```python
from build123d import *

# Parameters (mm, degrees)
F1_DEPTH = 8
F3_DEPTH = 25


with BuildPart() as f1:
    # F0 (on Top) → F1 (new body)
    with BuildSketch(Plane.XY):
        Polygon((20.7106781187, -50), (50, -20.7106781187), (50, 20.7106781187), (20.7106781187, 50), (-20.7106781187, 50), (-50, 20.7106781187), (-50, -20.7106781187), (-20.7106781187, -50), align=None)
    extrude(amount=F1_DEPTH)

    # F2 (on face) → F3 (cut)
    with BuildSketch(Plane.XY.offset(8)):
        with BuildLine():
            ThreePointArc((24.5349567524, 31.5917061451), (24.7489552671, 24.7485194141), (31.5921382283, 24.5344003832))
            ThreePointArc((31.5921382283, 24.5344003832), (28.2845203052, 28.2840221875), (24.5349567524, 31.5917061451))
        make_face()
        with BuildLine():
            ThreePointArc((24.5349567524, 31.5917061451), (28.2845203052, 28.2840221875), (31.5921382283, 24.5344003832))
            ThreePointArc((31.5921382283, 24.5344003832), (32.8418270546, 26.2270936053), (33.2845203052, 28.2840221875))
            ThreePointArc((33.2845203052, 28.2840221875), (30.052595846, 32.9609772741), (24.5349567524, 31.5917061451))
        make_face()
        with BuildLine():
            ThreePointArc((-4.9902248196, 39.6875), (0, 35), (4.9902248196, 39.6875))
            ThreePointArc((4.9902248196, 39.6875), (0, 40), (-4.9902248196, 39.6875))
        make_face()
        with BuildLine():
            ThreePointArc((-4.9902248196, 39.6875), (0, 40), (4.9902248196, 39.6875))
            ThreePointArc((4.9902248196, 39.6875), (4.9975556074, 39.8436735754), (5, 40))
            ThreePointArc((5, 40), (-0.1563264246, 44.9975556074), (-4.9902248196, 39.6875))
        make_face()
        with BuildLine():
            ThreePointArc((-31.5918062772, 24.5348278197), (-28.2841376224, 28.2844048719), (-24.5345293173, 31.5920380979))
            ThreePointArc((-24.5345293173, 31.5920380979), (-31.8196548252, 31.8199554809), (-31.5918062772, 24.5348278197))
        make_face()
        with BuildLine():
            ThreePointArc((-23.2841376224, 28.2844048719), (-23.607170575, 30.0524487732), (-24.5345293173, 31.5920380979))
            ThreePointArc((-24.5345293173, 31.5920380979), (-28.2841376224, 28.2844048719), (-31.5918062772, 24.5348278197))
            ThreePointArc((-31.5918062772, 24.5348278197), (-26.2272398702, 23.7270842076), (-23.2841376224, 28.2844048719))
        make_face()
        with BuildLine():
            ThreePointArc((-39.6875, -4.9902248196), (-40, 0), (-39.6875, 4.9902248196))
            ThreePointArc((-39.6875, 4.9902248196), (-45, 0), (-39.6875, -4.9902248196))
        make_face()
        with BuildLine():
            ThreePointArc((-35, 0), (-36.3556550657, 3.4232659844), (-39.6875, 4.9902248196))
            ThreePointArc((-39.6875, 4.9902248196), (-40, 0), (-39.6875, -4.9902248196))
            ThreePointArc((-39.6875, -4.9902248196), (-36.3556550657, -3.4232659844), (-35, 0))
        make_face()
        with BuildLine():
            ThreePointArc((-31.5921382283, -24.5344003832), (-31.8200853434, -31.8195249609), (-24.5349567524, -31.5917061451))
            ThreePointArc((-24.5349567524, -31.5917061451), (-28.2845203052, -28.2840221875), (-31.5921382283, -24.5344003832))
        make_face()
        with BuildLine():
            ThreePointArc((-31.5921382283, -24.5344003832), (-28.2845203052, -28.2840221875), (-24.5349567524, -31.5917061451))
            ThreePointArc((-24.5349567524, -31.5917061451), (-23.6075652186, -30.0520977283), (-23.2845203052, -28.2840221875))
            ThreePointArc((-23.2845203052, -28.2840221875), (-26.227591723, -23.7267154382), (-31.5921382283, -24.5344003832))
        make_face()
        with BuildLine():
            ThreePointArc((-4.9902248196, -39.6875), (0, -40), (4.9902248196, -39.6875))
            ThreePointArc((4.9902248196, -39.6875), (0, -35), (-4.9902248196, -39.6875))
        make_face()
        with BuildLine():
            ThreePointArc((5, -40), (4.9975556074, -39.8436735754), (4.9902248196, -39.6875))
            ThreePointArc((4.9902248196, -39.6875), (0, -40), (-4.9902248196, -39.6875))
            ThreePointArc((-4.9902248196, -39.6875), (-0.1563264246, -44.9975556074), (5, -40))
        make_face()
        with BuildLine():
            ThreePointArc((24.5344003832, -31.5921382283), (28.2840221875, -28.2845203052), (31.5917061451, -24.5349567524))
            ThreePointArc((31.5917061451, -24.5349567524), (24.7485194141, -24.7489552671), (24.5344003832, -31.5921382283))
        make_face()
        with BuildLine():
            ThreePointArc((33.2840221875, -28.2845203052), (32.8413470491, -26.2276318527), (31.5917061451, -24.5349567524))
            ThreePointArc((31.5917061451, -24.5349567524), (28.2840221875, -28.2845203052), (24.5344003832, -31.5921382283))
            ThreePointArc((24.5344003832, -31.5921382283), (30.052056545, -32.9614909605), (33.2840221875, -28.2845203052))
        make_face()
        with BuildLine():
            ThreePointArc((39.6875, -4.9902248196), (39.9217985567, -2.5), (40, 0))
            ThreePointArc((40, 0), (39.9217985567, 2.5), (39.6875, 4.9902248196))
            ThreePointArc((39.6875, 4.9902248196), (35, 0), (39.6875, -4.9902248196))
        make_face()
        with BuildLine():
            ThreePointArc((39.6875, 4.9902248196), (39.9217985567, 2.5), (40, 0))
            ThreePointArc((40, 0), (39.9217985567, -2.5), (39.6875, -4.9902248196))
            ThreePointArc((39.6875, -4.9902248196), (43.4232659844, -3.6443449343), (45, 0))
            ThreePointArc((45, 0), (43.4232659844, 3.6443449343), (39.6875, 4.9902248196))
        make_face()
    extrude(amount=-F3_DEPTH, mode=Mode.SUBTRACT)


solid = f1.part
```
Verification items for the finished model (mm, model axes). Round coordinates to 2 decimals unless told otherwise and drop trailing zeros. Loops run counter-clockwise (first coordinate to the right, second up) from the corner with the lowest first, then second, coordinate; pieces in that order, holes last. Notation, with made-up numbers: (25.5, 37) -> (68.5, 37) arc R5 cw to (68.5, 44) -> close; hole circle Ø6 at (89, 19.25). An arc over 180 degrees is marked (long way). Answer as a JSON object with one key per item and string values.
Q1. Go/stop test with a flat-tipped pin: P1, Ø2, axis at x = 19.5, y = 25, coming from the -Z side. Record where the tip stops, or that it passes through.
Data:
{"P1": "stops at z = 0"}
Q2. Section check C-C (z = 3). State how many separate pieces and enclosed holes the cut face has, then the cut area to 3 significant figures.
Data:
{"separate pieces": "1", "enclosed holes": "8", "area": "7,660 mm2"}
Q3. Draft check along X on faces 1 (the flat face through (-50, 0, 4)), 2 (the flat face through (0, -50, 4)), 3 (the flat face through (50, 0, 4)). Enter one of: pulls with the +X half, pulls with the -X half, needs draft (parallel to the pull), parting line crosses it, or undercut.
Data:
{"face 1": "pulls with the -X half", "face 2": "needs draft", "face 3": "pulls with the +X half"}
Q4. Section check A-A (x = 0). Record the boundary of the cut face in (y, z).
Data:
{"outline": "(-50, 0) -> (-45, 0) -> (-45, 8) -> (-50, 8) -> close; (-35, 0) -> (35, 0) -> (35, 8) -> (-35, 8) -> close; (45, 0) -> (50, 0) -> (50, 8) -> (45, 8) -> close"}
Q5. Section check D-D (x = -28.5). Record the boundary of the cut face in (y, z), then the cut area to 3 significant figures.
Data:
{"outline": "(-42.21, 0) -> (-33.28, 0) -> (-33.28, 8) -> (-42.21, 8) -> close; (-23.29, 0) -> (23.29, 0) -> (23.29, 8) -> (-23.29, 8) -> close; (33.28, 0) -> (42.21, 0) -> (42.21, 8) -> (33.28, 8) -> close", "area": "516 mm2"}
Q6. Section check B-B (y = 36.5). Record the boundary of the cut face in (x, z).
Data:
{"outline": "(-34.21, 0) -> (-3.57, 0) -> (-3.57, 8) -> (-34.21, 8) -> close; (3.57, 0) -> (34.21, 0) -> (34.21, 8) -> (3.57, 8) -> close"}
Q7. Scan lines: line 1 (Y direction, x = 28.5, z = 7.5); line 2 (X direction, y = -29.5, z = 6); line 3 (Y direction, x = -1, z = 0.5). Record each from-to range of solid material in increasing order. Write a range as from..to.
Data:
{"line 1": "y = -42.21..-33.28, -23.29..23.29, 33.28..42.21", "line 2": "x = -41.21..-33.13, -23.43..23.43, 33.13..41.21", "line 3": "y = -50..-44.9, -35.1..35.1, 44.9..50"}
